Model file for the job. Use its own axes, mm. A direction names the side the tool comes from. Round coordinates to 2 decimals unless told otherwise and drop trailing zeros. Write each loop counter-clockwise with the first axis right and the second up, starting at its lowest first coordinate (ties: lowest second). Pieces come first, ordered by that corner, then holes. Notation, with made-up numbers: (7, -2) - (46, -2) arc R12 cw to (46, 12) - close; hole circle Ø9 at (53, 68.25). An arc over 180 degrees is marked (long way). One line per item, written item: value.
from build123d import *

# Parameters (mm, degrees)
SKETCH1_R           = 1.25
BOSS_EXTRUDE1_DEPTH = 0.75
FILLET1_R           = 1.5


with BuildPart() as part:
    # Sketch1 → Boss-Extrude1 (new, symmetric)
    with BuildSketch(Plane.XY):
        with BuildLine():
            Line((7.097768331, 17.408666943), (5.091491735, 14.047621322))
            ThreePointArc((5.091491735, 14.047621322), (6.070373947, 10.169487005), (9.948508265, 11.148369217))
            Line((9.948508265, 11.148369217), (11.028531075, 12.957693985))
            ThreePointArc((11.028531075, 12.957693985), (0, -15.918193069), (-11.028531075, 12.957693985))
            Line((-11.028531075, 12.957693985), (-9.948508265, 11.148369217))
            ThreePointArc((-9.948508265, 11.148369217), (-6.070373947, 10.169487005), (-5.091491735, 14.047621322))
            Line((-5.091491735, 14.047621322), (-7.097768331, 17.408666943))
            ThreePointArc((-7.097768331, 17.408666943), (0, -18.8), (7.097768331, 17.408666943))
        make_face()
        with Locations(Location((-7.52, 12.59799527, 0), (0, 0, 180))):
            Circle(SKETCH1_R, mode=Mode.SUBTRACT)
        with Locations((7.52, 12.59799527)):
            Circle(SKETCH1_R, mode=Mode.SUBTRACT)
    extrude(amount=BOSS_EXTRUDE1_DEPTH, both=True)

    # Fillet1
    fillet1_edges = [part.edges().sort_by_distance(p)[0] for p in [
        (-11.028531075, 12.957693985, 0),
        (11.028531075, 12.957693985, 0),
    ]]
    fillet(fillet1_edges, radius=FILLET1_R)


solid = part.part
1. Drop a flat-ended pin along its axis: pin 1 (2 mm diameter, centred on x = 7.52, y = 12.6, fed in from -Z). Give the stop position or say it passes through.
Report:
pin 1: through
2. Band-saw the part on A-A on y = 15. Write the cut outline in (x, z).
Report:
outline: (-11.33, -0.75) - (-5.66, -0.75) - (-5.66, 0.75) - (-11.33, 0.75) - close; (5.66, -0.75) - (11.33, -0.75) - (11.33, 0.75) - (5.66, 0.75) - close
3. Wall check: probe 1 along X at (y, z) = (10, 0.4); probe 2 along X at (y, z) = (11.5, -0.55); probe 3 along Y at (x, z) = (7.52, -0.2). Give the ranges that are in metal, low to high. Write a range as [from, to].
Report:
probe 1: [-15.92, -13.63], [-8.64, -6.4], [6.4, 8.64], [13.63, 15.92]
probe 2: [-14.87, -12.47], [-10.18, -8.12], [-6.92, -4.91], [4.91, 6.92], [8.12, 10.18], [12.47, 14.87]
probe 3: [-17.23, -14.11], [9.77, 11.35], [13.85, 17.23]
4. Mould opens along Y. For faces 1 (the face through (8.1, 11.49, -0.01)), 2 (the face through (-6.08, 15.7, 0.01)), 3 (the face through (8, 10, 0.75)) say: released by +Y, released by -Y, zero draft, split by the parting line, or undercut.
Report:
face 1: undercut
face 2: released by +Y
face 3: zero draft
5. Band-saw the part on B-B on x = 7.52. Write the cut outline in (y, z), plus the area to 3 significant figures.
Report:
outline: (-17.23, -0.75) - (-14.11, -0.75) - (-14.11, 0.75) - (-17.23, 0.75) - close; (9.77, -0.75) - (11.35, -0.75) - (11.35, 0.75) - (9.77, 0.75) - close; (13.85, -0.75) - (17.23, -0.75) - (17.23, 0.75) - (13.85, 0.75) - close
area: 12.1 mm²
6. Band-saw the part on D-D on x = 16. Write the cut outline in (y, z).
Report:
outline: (-9.87, -0.75) - (-3.58, -0.75) - (-3.58, 0.75) - (-9.87, 0.75) - close; (4.83, -0.75) - (9.87, -0.75) - (9.87, 0.75) - (4.83, 0.75) - close
7. Tool access for faces 4 (the face through (-11.17, 12.02, 0.01)), 5 (the face through (6.11, 15.75, 0.01)), 6 (the face through (8, 10, -0.75)): list every direction of +Z, -Z, +X, -X, +Y, -Y with a clear straight run to the whole face (end or side of a thin tool).
Report:
face 4: +Z, -Z
face 5: +Z, -Z, +Y
face 6: -Z, +X, -X, +Y, -Y
8. Band-saw the part on C-C on z = 0.35. Write the cut outline in (x, y), plus the area to 3 significant figures.
Report:
outline: (-12.45, 11.52) arc R1.5 cw to (-10.04, 11.3) - (-9.95, 11.15) arc R2.83 ccw to (-5.09, 14.05) - (-7.1, 17.41) arc R18.8 ccw (long way) to (7.1, 17.41) - (5.09, 14.05) arc R2.83 ccw to (9.95, 11.15) - (10.04, 11.3) arc R1.5 cw to (12.45, 11.52) arc R16.54 cw (long way) to start; hole circle Ø2.5 at (-7.52, 12.6); hole circle Ø2.5 at (7.52, 12.6)
area: 271 mm²
